```python
from build123d import *

# Parameters (mm, degrees)
SKETCH1_W                     = 41.91
SKETCH1_H                     = 38.1
BOSS_EXTRUDE1_DEPTH           = 5.08
TAP_DRILL_FOR_4_48_TAP1_D     = 2.3749
TAP_DRILL_FOR_4_48_TAP1_DEPTH = 10.16
TAP_DRILL_FOR_4_48_TAP1_TIP   = 0.713491942


with BuildPart() as part:
    # Sketch1 → Boss-Extrude1 (new body)
    with BuildSketch(Plane(origin=(0, 0, 0), x_dir=(1, 0, 0), z_dir=(0, 1, 0))):
        with Locations((-4.30427027, -8.5725)):
            Rectangle(SKETCH1_W, SKETCH1_H)
    extrude(amount=BOSS_EXTRUDE1_DEPTH)

    # Tap Drill for #4-48 Tap1
    with Locations(Plane.ZY.offset(25.25927027)):
        with Locations((-0.3175, 2.422722957), (22.5425, 2.422722957)):
            Hole(TAP_DRILL_FOR_4_48_TAP1_D / 2, depth=TAP_DRILL_FOR_4_48_TAP1_DEPTH)
            with Locations((0, 0, -(TAP_DRILL_FOR_4_48_TAP1_DEPTH + TAP_DRILL_FOR_4_48_TAP1_TIP / 2))):  # 118° drill point
                Cone(0, TAP_DRILL_FOR_4_48_TAP1_D / 2, TAP_DRILL_FOR_4_48_TAP1_TIP, mode=Mode.SUBTRACT)


solid = part.part
```
Geometry: final body of the model. Coordinates: model frame, mm. A direction names the side the tool comes from. Give positions to 0.01 mm unless a question says otherwise; leave off trailing zeros. Loops run counter-clockwise (first coordinate to the right, second up) from the corner with the lowest first, then second, coordinate; pieces in that order, holes last. Notation, with made-up numbers: (35.5, 1) - (72.5, 1) arc R14 ccw to (72.5, 9) - close; hole circle Ø8 at (68, 37.25). An arc over 180 degrees is marked (long way). Answer as CSV lines item,"result". Start each with the question number.
(1) Reachability of faces 5 (the face through (-5, 3, -10.478)), 6 (the face through (-20.11, 2.78, 21.41)) from +Z, -Z, +X, -X, +Y, -Y: full face, straight path, thin tool, end or side. Return the list, or none.
(2) Pin query (flat end, axial travel): P1, Ø5, axis at x = -14, z = -1, coming from the -Y side; P2, Ø1.4, axis at y = 2.42, z = 22.54, coming from the -X side. Return the tip coordinate at first contact, or that it passes through.
(3) Ray query, line 1 along Z through (x, y) = (-19, 2.55); line 2 along X through (y, z) = (2.4, -1). Return the intervals inside material, ascending. Write a range as [from, to].
(4) Mould query, pull axis Y, two halves, no side actions, for faces 1 (the face through (-5, 5.08, 8)), 2 (the face through (-14.51, 2.48, 22.74)), 3 (the face through (-20.11, 3.6, -0.16)), 4 (the face through (-5, 3, 27.623)). Classes: +Y half, -Y half, draft (parallel to the pull), parting line (faces both ways), or undercut.
(5) Section query A-A (x = -16.5). Output: boundary loops of the cut face in (y, z).
Worked answers:
1,face 5,"-Z, +X, -X, +Y, -Y"
1,face 6,"-X"
2,P1,"stops at y = 0"
2,P2,"stops at x = -14.81"
3,line 1,"z = [-10.48, -1.5], [0.86, 21.36], [23.72, 27.62]"
3,line 2,"x = [-14.8, 16.65]"
4,face 1,"+Y half"
4,face 2,"undercut"
4,face 3,"undercut"
4,face 4,"draft"
5,outline,"(0, -10.48) - (5.08, -10.48) - (5.08, 27.62) - (0, 27.62) - close; hole circle Ø2.37 at (2.42, -0.32); hole circle Ø2.37 at (2.42, 22.54)"
